Work out the finished part from the listing and answer in its coordinate system (mm). Give positions to 0.01 mm unless a question says otherwise; leave off trailing zeros. Order: outer loops, then holes, each group sorted by start corner. A loop starts at its lowest first (then second) coordinate and runs counter-clockwise, first axis right, second up. Notation, with made-up numbers: M 38,64.5 L 95,64.5 A31 ccw 95,91.5 Z; hole C 88.5,24 d10. An arc over 180 degrees is marked long. One line per item, written item: value.
from build123d import *

# Parameters (mm, degrees)
F0_W     = 12.7
F0_H     = 12.7
F1_DEPTH = 12.7


# Not quite as in the source:
# - ends of sketch curves that miss each other by under 0.0002 mm in the source are joined
# - a feature names something its author has since deleted; it is built from what else it names


with BuildPart() as f1:
    # F0 (on Top) → F1 (new body)
    with BuildSketch(Plane.XY):
        Polygon((-112.6111072004, 68.7462910332), (-125.3111072004, 68.7462910332), (-125.3111072004, 56.0462910332), (-138.0111072004, 56.0462921858), (-138.0111072004, 43.3462910332), (-138.0111072004, 30.6462910332), (-138.0111072004, 17.9462910332), (-138.0111072004, 5.2462910332), (-138.0111072004, -7.4537089668), (-138.0111072004, -20.1537089668), (-138.0111072004, -32.8537089668), (-138.0111072004, -45.5537089668), (-138.0111072004, -58.2537089668), (-125.3111072004, -58.2537089668), (-125.3111072004, -45.5537089668), (-112.6111072004, -45.5537089668), (-112.6111072004, -58.2537089668), (-99.9111072004, -58.2537089668), (-99.9111072004, -45.5537089668), (-87.2111072004, -45.5537089668), (-87.2111072004, -58.2537089668), (-74.5111072004, -58.2537089668), (-74.5111072004, -45.5537089668), (-61.8111072004, -45.5537089668), (-61.8111072004, -58.2537089668), (-49.1111072004, -58.2537089668), (-49.1111072004, -45.5537089668), (-36.4111072004, -45.5537089668), (-36.4111072004, -58.2537089668), (-23.7111072004, -58.2537089668), (-23.7111072004, -45.5537089668), (-11.0111072004, -45.5537089668), (-11.0111072004, -58.2537089668), (1.6888927996, -58.2537089668), (1.6888927996, -45.5537089668), (14.3888927996, -45.5537089668), (14.3888927996, -58.2537089668), (27.0888927996, -58.2537089668), (27.0888927996, -45.5537089668), (39.7888927996, -45.5537089668), (39.7888927996, -58.2537089668), (52.4888927996, -58.2537089668), (52.4888927996, -45.5537089668), (65.1888927996, -45.5537089668), (65.1888927996, -58.2537089668), (77.8888927996, -58.2537089668), (77.8888927996, -45.5537089668), (90.5888927996, -45.5537089668), (90.5888927996, -58.2537089668), (103.2888927996, -58.2537089668), (103.2888927996, -45.5537089668), (115.9888927996, -45.5537089668), (115.9888927996, -58.2537089668), (128.6888927996, -58.2537089668), (128.6888927996, -45.5537089668), (141.3888927996, -45.5537089668), (141.3888927996, -58.2537089668), (154.0888927996, -58.2537089668), (154.0888927996, -45.5537089668), (166.7888927996, -45.5537089668), (166.7888927996, -58.2537089668), (179.4888927996, -58.2537089668), (179.4888927996, -45.5537089668), (192.1888927996, -45.5537089668), (192.1888927996, -58.2537089668), (204.8888927996, -58.2537089668), (204.8888927996, -45.5537089668), (217.5888927996, -45.5537089668), (217.5888927996, -58.2537089668), (230.2888927996, -58.2537089668), (230.2888927996, -45.5537089668), (242.9888927996, -45.5537089668), (242.9888927996, -32.8537103117), (242.9888927996, -20.1537098634), (242.9888927996, -7.4537103117), (242.9888927996, 5.2462896883), (242.9888927996, 17.9462896883), (242.9888927996, 30.6462901366), (242.9888927996, 43.3462896883), (242.9888927996, 56.0462905208), (242.9888927996, 68.7462910332), (230.2888927996, 68.7462910332), (230.2888927996, 56.0462921858), (217.5888927996, 56.0462921858), (217.5888927996, 68.7462921858), (204.8888927996, 68.7462910332), (204.8888927996, 56.0462921858), (192.1888927996, 56.0462921858), (192.1888927996, 68.7462910332), (179.4888927996, 68.7462910332), (179.4888927996, 56.0462921858), (166.7888927996, 56.0462921858), (166.7888927996, 68.7462921858), (154.0888927996, 68.7462910332), (154.0888927996, 56.0462921858), (141.3888927996, 56.0462921858), (141.3888927996, 68.7462910332), (128.6888927996, 68.7462910332), (128.6888927996, 56.0462921858), (115.9888927996, 56.0462921858), (115.9888927996, 68.7462921858), (103.2888927996, 68.7462910332), (103.2888927996, 56.0462921858), (90.5888927996, 56.0462921858), (90.5888927996, 68.7462921858), (77.8888927996, 68.7462910332), (77.8888927996, 56.0462921858), (65.1888927996, 56.0462921858), (65.1888927996, 68.7462921858), (52.4888927996, 68.7462910332), (52.4888927996, 56.0462921858), (39.7888927996, 56.0462921858), (39.7888927996, 68.7462921858), (27.0888927996, 68.7462910332), (27.0888927996, 56.0462921858), (14.3888927996, 56.0462921858), (14.3888927996, 68.7462921858), (1.6888927996, 68.7462910332), (1.6888927996, 56.0462921858), (-11.0111072004, 56.0462921858), (-11.0111072004, 68.7462921858), (-23.7111072004, 68.7462910332), (-23.7111072004, 56.0462921858), (-36.4111072004, 56.0462921858), (-36.4111072004, 68.7462921858), (-49.1111072004, 68.7462910332), (-49.1111072004, 56.0462921858), (-61.8111072004, 56.0462921858), (-61.8111072004, 68.7462921858), (-74.5111072004, 68.7462910332), (-74.5111072004, 56.0462921858), (-87.2111072004, 56.0462921858), (-87.2111072004, 68.7462921858), (-99.9111072004, 68.7462910332), (-99.9111072004, 56.0462921858), (-112.6111072004, 56.0462921858), align=None)
        with Locations((-144.3611072004, -51.9037089668)):
            Rectangle(F0_W, F0_H)
        Polygon((-138.0111072004, 43.3462910332), (-138.0111072004, 56.0462916095), (-150.7111072004, 56.0462910332), (-150.7111072004, 43.3462910332), align=None)
        with Locations((-144.3611072004, 24.2962910332)):
            Rectangle(F0_W, F0_H)
        with Locations((-144.3611072004, -1.1037089668)):
            Rectangle(F0_W, F0_H)
        with Locations((-144.3611072004, -26.5037089668)):
            Rectangle(F0_W, F0_H)
        with Locations((249.3388927996, -39.2037103117)):
            Rectangle(F0_W, F0_H)
        with Locations((249.3388927996, -13.8037103117)):
            Rectangle(F0_W, F0_H)
        with Locations((249.3388927996, 11.5962896883)):
            Rectangle(F0_W, F0_H)
        with Locations((249.3388927996, 36.9962896883)):
            Rectangle(F0_W, F0_H)
        Polygon((255.6888927996, 68.7462896883), (242.9888927996, 68.7462896883), (242.9888927996, 56.0462905208), (255.6888927996, 56.0462896883), align=None)
    extrude(amount=F1_DEPTH)


solid = f1.part
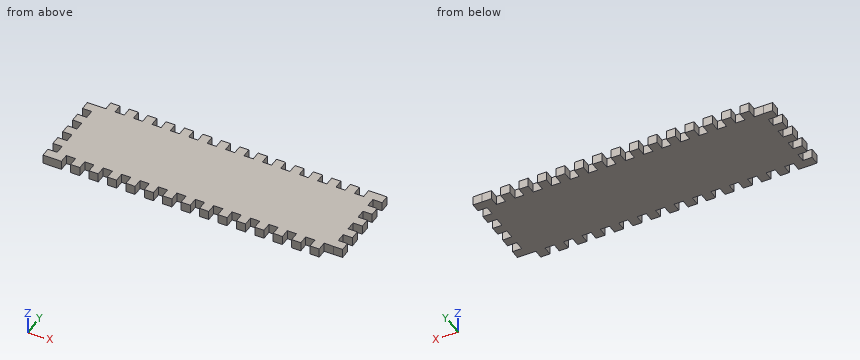
(1) Given P1, Ø4, axis at y = -2.5, z = 6, coming from the +X side; P2, Ø4, axis at x = -44, z = 4, coming from the -Y side; P3, Ø6.5, axis at y = -42, z = 9, coming from the -X side, each flat-ended and moving along its own axis, determine where each tip first touches the part or whether it passes through.
Findings:
P1: stops at x = 242.99
P2: stops at y = -45.55
P3: stops at x = -138.01
(2) Section B-B, the plane y = -37.5 is taken. Give the vertices of the cut face in (x, z).
Findings:
outline: M -138.01,0 L 255.69,0 L 255.69,12.7 L -138.01,12.7 Z
(3) Find the intervals of material crossed by probe 1 along Y at (x, z) = (-14.5, 4); probe 2 along Y at (x, z) = (-2.5, 9.25); probe 3 along X at (y, z) = (-17, 2), in increasing order. Write a range as from..to.
Findings:
probe 1: y = -45.55..68.75
probe 2: y = -58.25..56.05
probe 3: x = -138.01..255.69
(4) Section A-A, the plane x = -53 is taken. Give the vertices of the cut face in (y, z), then the cut area to 3 significant figures.
Findings:
outline: M -58.25,0 L 56.05,0 L 56.05,12.7 L -58.25,12.7 Z
area: 1,450 mm^2
